```python
from build123d import *

# Parameters (mm, degrees)
BOSS_EXTRUDE1_DEPTH     = 11.5
SKETCH2_OUTSIDE_W       = 84.912
SKETCH2_OUTSIDE_H       = 140.162
CUT_EXTRUDE2_DEPTH      = 7.5
CUT_EXTRUDE3_DEPTH      = 129.307516771
CUT_EXTRUDE3_DEPTH_BACK = 129.307516771
SKETCH4_R               = 1.75
SKETCH5_W               = 57.250055546
SKETCH5_H               = 43
BOSS_EXTRUDE2_DEPTH     = 4
SKETCH6_R               = 1.75
CUT_EXTRUDE4_DEPTH      = 129.047135306
FILLET1_R               = 3


with BuildPart() as part:
    # Sketch1 → Boss-Extrude1 (new, symmetric)
    with BuildSketch(Plane.XY):
        Polygon((0, 0), (57.250055546, 0), (57.250055546, 15), (24.066011022, 34.158817039), (46.210390637, 95), (57.250055546, 112.5), (52.250055546, 112.5), (18.50330035, 81.314771653), (0, 45), align=None)
    extrude(amount=BOSS_EXTRUDE1_DEPTH, both=True)

    # Sketch2 outside → Cut-Extrude2 (cut, symmetric)
    with BuildSketch(Plane.XY):
        with Locations((28.625, 56.25)):
            Rectangle(SKETCH2_OUTSIDE_W, SKETCH2_OUTSIDE_H)
        Polygon((21.742887775, 78.862062909), (4, 44.039684964), (4, 24.475940791), (57.250055546, 6.97368477), (57.250055546, 0), (0, 0), (0, 45), (18.50330035, 81.314771653), (52.250055546, 112.5), (57.250055546, 112.5), (47.787485624, 97.5), (47.787485624, 102.92976146), align=None, mode=Mode.SUBTRACT)
    extrude(amount=CUT_EXTRUDE2_DEPTH, both=True, mode=Mode.SUBTRACT)

    # Sketch4 → Cut-Extrude3 (cut, two sides: drawn at the far end of the back side and taken through both)
    with BuildSketch(Plane.XY.offset(11.5).offset(-CUT_EXTRUDE3_DEPTH_BACK)):
        with Locations((45.250055546, 16.444166257)):
            Circle(SKETCH4_R)
        with Locations((31.000040397, 21.127868666)):
            Circle(SKETCH4_R)
        with Locations((16.750025248, 25.811571075)):
            Circle(SKETCH4_R)
    extrude(amount=CUT_EXTRUDE3_DEPTH + CUT_EXTRUDE3_DEPTH_BACK, mode=Mode.SUBTRACT)

    # Sketch5 → Boss-Extrude2 (add)
    with BuildSketch(Plane.XZ):
        with Locations((28.625027773, 0)):
            Rectangle(SKETCH5_W, SKETCH5_H)
    extrude(amount=BOSS_EXTRUDE2_DEPTH)

    # Sketch6 → Cut-Extrude4 (cut, symmetric)
    with BuildSketch(Plane(origin=(0, 0, 0), x_dir=(1, 0, 0), z_dir=(0, 1, 0))):
        with Locations(Location((7.250055546, 18, 0), (0, 0, 270))):
            Circle(SKETCH6_R)
        with Locations(Location((47.250055546, 18, 0), (0, 0, 270))):
            Circle(SKETCH6_R)
    cut_extrude4 = extrude(amount=CUT_EXTRUDE4_DEPTH, both=True, mode=Mode.SUBTRACT)

    # Mirror5: Cut-Extrude4 across plane
    add(cut_extrude4.mirror(Plane.XY), mode=Mode.SUBTRACT)

    # Fillet1
    fillet1_edges = [part.edges().sort_by_distance(p)[0] for p in [
        (28.625027773, 0, -11.5),
        (28.625027773, 0, 11.5),
    ]]
    fillet(fillet1_edges, radius=FILLET1_R)


solid = part.part
```
Work out the finished part from the listing and answer in its coordinate system (mm). A direction names the side the tool comes from. Give positions to 0.01 mm unless a question says otherwise; leave off trailing zeros. Loops run counter-clockwise (first coordinate to the right, second up) from the corner with the lowest first, then second, coordinate; pieces in that order, holes last. Notation, with made-up numbers: (27, -3) - (31, -3) arc R30 ccw to (31, 24) - close; hole circle Ø4 at (-17, -24.5). An arc over 180 degrees is marked (long way). Use CSV: the item, a comma, the result in double quotes. Start each with the question number.
(1) Determine the mould class of faces 5 (the face through (28, -2, 21.5)), 6 (the face through (43.96, 17.627, -9.528)), 7 (the face through (4, 34, 0)), 8 (the face through (27, 48, 7.5)) for opening direction Z: released by +Z, released by -Z, zero draft, split by the parting line, or undercut.
(2) Find section C-C, the plane y = 72.5. Determine the outline of the cut face in (x, z), plus the area to 3 significant figures.
(3) A tool of negligible diameter and unlimited length cuts with its end or side. For faces 1 (the face through (47.787, 100, 0)), 2 (the face through (35, 64.2, 9.5)), 3 (the face through (28, 0, -18)), 4 (the face through (0, 21, 0)), from which of +Z, -Z, +X, -X, +Y, -Y can it reach the whole face along a straight path? Write none if from no direction.
(4) Find the intervals of material crossed by L1, parallel to X at y = -1.2, z = -18; L2, parallel to Y at x = 41, z = 4.5; L3, parallel to Y at x = 46.5, z = 14.5, in increasing order.
(5) Find section A-A, the plane z = 18. Determine the outline of the cut face in (x, y).
(6) Each of these flat-tipped pins is pushed along its axis until it touches: pin 1 (17 mm diameter, centred on x = 23.5, y = 50.5, fed in from -Z); pin 2 (16 mm diameter, centred on x = 33.5, y = 69, fed in from +Z); pin 3 (5.5 mm diameter, centred on x = 30.5, z = 18.5, fed in from +Y); pin 4 (3 mm diameter, centred on x = 16.75, y = 25.81, fed in from +Z). Where does it stop, or does it pass through?
(7) Find section D-D, the plane y = 13. Determine the outline of the cut face in (x, z), plus the area to 3 significant figures.
(8) Find section B-B, the plane x = 36. Determine the outline of the cut face in (y, z), plus the area to 3 significant figures.
Results found:
1,face 5,"released by +Z"
1,face 6,"zero draft"
1,face 7,"undercut"
1,face 8,"undercut"
2,outline,"(14.01, -11.5) - (38.02, -11.5) - (38.02, -7.5) - (18.5, -7.5) - (18.5, 7.5) - (38.02, 7.5) - (38.02, 11.5) - (14.01, 11.5) - close"
2,area,"259 mm^2"
3,face 1,"none"
3,face 2,"+Z, -Z, +X"
3,face 3,"-Z, +X, -X, +Y"
3,face 4,"+Z, -Z, -X, +Y, -Y"
4,L1,"0 to 5.5, 9 to 45.5, 49 to 57.25"
4,L2,"-4 to 12.31, 96.66 to 102.1"
4,L3,"-4 to 0"
5,outline,"(0, -4) - (5.5, -4) - (5.5, 0) - (0, 0) - close; (9, -4) - (45.5, -4) - (45.5, 0) - (9, 0) - close; (49, -4) - (57.25, -4) - (57.25, 0) - (49, 0) - close"
6,pin 1,"z = -11.5"
6,pin 2,"z = 11.5"
6,pin 3,"y = 0"
6,pin 4,"through"
7,outline,"(0, -11.5) - (57.25, -11.5) - (57.25, -7.5) - (38.92, -7.5) - (38.92, 7.5) - (57.25, 7.5) - (57.25, 11.5) - (0, 11.5) - close"
7,area,"1,040 mm^2"
8,outline,"(-4, -21.5) - (0, -21.5) - (0, -14.5) arc R3 cw to (3, -11.5) - (27.27, -11.5) - (27.27, -7.5) - (13.96, -7.5) - (13.96, 7.5) - (27.27, 7.5) - (27.27, 11.5) - (3, 11.5) arc R3 cw to (0, 14.5) - (0, 21.5) - (-4, 21.5) - close; (66.95, -11.5) - (97.48, -11.5) - (97.48, 11.5) - (66.95, 11.5) - (66.95, 7.5) - (92.04, 7.5) - (92.04, -7.5) - (66.95, -7.5) - close"
8,area,"929 mm^2"
